Autodesk Inventor part; units mm, degrees
ref_plane "YZ Plane" through (0, 0, 0) normal (1, 0, 0) x (0, 1, 0)
ref_plane "XZ Plane" through (0, 0, 0) normal (0, 1, 0) x (-1, 0, 0)
ref_plane "XY Plane" through (0, 0, 0) normal (0, 0, 1) x (1, 0, 0)
sketch "Sketch1" plane through (0, 0, 0) normal (0, 1, 0) x (-1, 0, 0)
  line L0 (0, 0) -> (105.41, 0)
  line L1 (105.41, 0) -> (105.41, 863.6)
  line L2 (105.41, 863.6) -> (0, 863.6)
  line L3 (0, 863.6) -> (0, 0)
  dimension "d0" = 105.41
  dimension "d1" = 863.6
extrude "Extrusion1" add sketch "Sketch1" along normal blind 12.7
sketch "Sketch2" plane through (0, 12.7, 0) normal (0, 1, 0) x (1, 0, 0)
  line L0 (0, 0) -> (-105.41, 0)
  line L1 (0, 0) -> (-12.7, 0)
  line L2 (-12.7, 0) -> (-12.7, 12.7)
  line L3 (-12.7, 12.7) -> (0, 12.7)
  line L4 (0, 12.7) -> (0, 0)
  line L5 (-105.41, 0) -> (-105.41, -863.6)
  line L6 (0, 12.7) -> (-105.41, 12.7)
  line L7 (-105.41, 12.7) -> (-105.41, 0)
  line L8 (-105.41, 0) -> (0, 0)
  line L9 (0, 0) -> (0, 12.7)
  line L10 (0, -863.6) -> (0, 0)
  line L11 (0, -863.6) -> (-105.41, -863.6)
  line L12 (-105.41, -863.6) -> (-105.41, -876.3)
  line L13 (-105.41, -876.3) -> (0, -876.3)
  line L14 (0, -876.3) -> (0, -863.6)
  line L15 (-105.41, -863.6) -> (-92.71, -863.6)
  line L16 (-92.71, -863.6) -> (-92.71, 12.7)
  line L17 (-92.71, 12.7) -> (-105.41, 12.7)
  line L18 (-105.41, 12.7) -> (-105.41, -863.6)
  line L19 (0, 12.7) -> (-12.7, 12.7)
  line L20 (-12.7, 12.7) -> (-12.7, -876.3)
  line L21 (-12.7, -876.3) -> (0, -876.3)
  line L22 (0, -876.3) -> (0, 12.7)
  point P0 (-12.7, -863.6)
  point P1 (-92.71, 0)
  dimension "d4" = 12.7
  dimension "d5" = 12.7
  dimension "d6" = 12.7
  dimension "d7" = 12.7
  dimension "d8" = 12.7
extrude "Extrusion2" add sketch "Sketch2" along normal blind 95.25 and the other way blind 12.7 contours L10 L11 L20 L0 | L0 L2 L3 L4 | L0 L16 L6 L2 | L14 L13 L20 L11 | L16 L11 L5 L0 | L0 L7 L6 L16 | L20 L13 L12 L11
sketch "Sketch3" plane through (-105.41, 107.95, 876.3) normal (0, 0, 1) x (1, 0, 0)
  line L0 (12.7, -95.25) -> (92.71, -95.25)
  line L1 (12.7, -95.25) -> (12.7, 0)
  line L2 (92.71, -95.25) -> (92.71, 0)
  line L3 (92.71, -95.25) -> (77.47, -95.25)
  line L4 (77.47, -95.25) -> (77.47, -12.7)
  line L5 (77.47, -12.7) -> (92.71, -12.7)
  line L6 (92.71, -12.7) -> (92.71, -95.25)
  line L7 (12.7, -95.25) -> (27.94, -95.25)
  line L8 (27.94, -95.25) -> (27.94, -12.7)
  line L9 (27.94, -12.7) -> (12.7, -12.7)
  line L10 (12.7, -12.7) -> (12.7, -95.25)
  line L11 (27.94, -95.25) -> (34.29, -95.25)
  line L12 (34.29, -95.25) -> (34.29, -12.7)
  line L13 (34.29, -12.7) -> (27.94, -12.7)
  line L14 (27.94, -12.7) -> (27.94, -95.25)
  line L15 (77.47, -95.25) -> (71.12, -95.25)
  line L16 (71.12, -95.25) -> (71.12, -12.7)
  line L17 (71.12, -12.7) -> (77.47, -12.7)
  line L18 (77.47, -12.7) -> (77.47, -95.25)
  line L19 (34.29, -95.25) -> (49.53, -95.25)
  line L20 (49.53, -95.25) -> (49.53, -12.7)
  line L21 (49.53, -12.7) -> (34.29, -12.7)
  line L22 (34.29, -12.7) -> (34.29, -95.25)
  line L23 (71.12, -95.25) -> (55.88, -95.25)
  line L24 (55.88, -95.25) -> (55.88, -12.7)
  line L25 (55.88, -12.7) -> (71.12, -12.7)
  line L26 (71.12, -12.7) -> (71.12, -95.25)
  point P0 (105.41, -107.95)
  dimension "d13" = 15.24
  dimension "d14" = 82.55
  dimension "d15" = 15.24
  dimension "d16" = 6.35
  dimension "d17" = 6.35
  dimension "d18" = 15.24
  dimension "d19" = 15.24
extrude "Extrusion3" cut sketch "Sketch3" against normal blind 95.25 contours L1 L9 L8 L0 | L24 L25 L16 L0 | L12 L21 L20 L0 | L4 L5 L2 L0
sketch "Sketch5" plane through (-105.41, 107.95, 876.3) normal (0, 0, 1) x (1, 0, 0)
  line L0 (71.12, -95.25) -> (55.88, -95.25)
  line L1 (55.88, -95.25) -> (55.88, -12.7)
  line L2 (55.88, -12.7) -> (71.12, -12.7)
  line L3 (71.12, -12.7) -> (71.12, -95.25)
  line L4 (49.53, -95.25) -> (34.29, -95.25)
  line L5 (34.29, -95.25) -> (34.29, -12.7)
  line L6 (34.29, -12.7) -> (49.53, -12.7)
  line L7 (49.53, -12.7) -> (49.53, -95.25)
  line L8 (92.71, -95.25) -> (77.47, -95.25)
  line L9 (77.47, -95.25) -> (77.47, -12.7)
  line L10 (77.47, -12.7) -> (92.71, -12.7)
  line L11 (92.71, -12.7) -> (92.71, -95.25)
  line L12 (27.94, -95.25) -> (12.7, -95.25)
  line L13 (12.7, -95.25) -> (12.7, -12.7)
  line L14 (12.7, -12.7) -> (27.94, -12.7)
  line L15 (27.94, -12.7) -> (27.94, -95.25)
  line L16 (105.41, -107.95) -> (105.41, 0)
  line L17 (0, 0) -> (105.41, 0)
  line L18 (0, -107.95) -> (0, 0)
  line L19 (105.41, -107.95) -> (0, -107.95)
  line L20 (92.71, 0) -> (12.7, 0)
  circle A0 centre (52.705, 26.3525) radius 26.3525
  dimension "d40" = 52.705
extrude "Extrusion4" add sketch "Sketch5" against normal blind 1270 contours A0
sketch "Sketch6" plane through (0, 0, -12.7) normal (1, 0, 0) x (0, 0, -1)
  line L0 (0, 0) -> (-889, 0)
  line L1 (-444.5, 0) -> (-444.5, 160.655)
  line L2 (-889, 160.655) -> (381, 160.655)
  line L3 (-444.5, 160.655) -> (-444.5, 167.005)
  line L4 (-444.5, 0) -> (-444.5, -6.35)
  line L5 (-444.5, 167.005) -> (-428.625, 167.005)
  line L6 (-428.625, 167.005) -> (-460.375, 167.005)
  line L7 (-428.625, 167.005) -> (-460.375, 167.005)
  line L8 (-460.375, 167.005) -> (-460.375, -6.35)
  line L9 (-460.375, -6.35) -> (-428.625, -6.35)
  line L10 (-428.625, -6.35) -> (-428.625, 167.005)
  line L11 (-889, 0) -> (-793.75, 0)
  line L12 (0, 107.95) -> (0, 0)
  line L13 (0, 0) -> (-95.25, 0)
  line L14 (-95.25, 0) -> (-95.25, -6.35)
  line L15 (-793.75, 0) -> (-793.75, -6.35)
  line L16 (-793.75, -6.35) -> (-762, -6.35)
  line L17 (-762, -6.35) -> (-762, 167.005)
  line L18 (-762, 167.005) -> (-793.75, 167.005)
  line L19 (-793.75, 167.005) -> (-793.75, -6.35)
  line L20 (-95.25, -6.35) -> (-127, -6.35)
  line L21 (-127, -6.35) -> (-127, 167.005)
  line L22 (-127, 167.005) -> (-95.25, 167.005)
  line L23 (-95.25, 167.005) -> (-95.25, -6.35)
  line L24 (-111.125, 167.005) -> (-111.125, -6.35)
  line L25 (-777.875, -6.35) -> (-777.875, 167.005)
  line L26 (-777.875, 79.2503) -> (-762, 79.2503)
  line L27 (-111.125, 68.9503) -> (-95.25, 68.9503)
  line L28 (-451.8389, 167.005) -> (-451.8389, 163.0426)
  circle A0 centre (-444.5, 148.7424) radius 10.8761
  circle A1 centre (-444.5, 11.9126) radius 11.9126
  line L29 (-456.4123, 12.0028) -> (-455.3758, 148.8248)
  line L30 (-433.6242, 148.8248) -> (-432.5877, 12.0028)
  line L31 (-127, 12.7) -> (-139.7, 12.7)
  line L32 (-139.7, 12.7) -> (-165.1, 12.7)
  line L33 (-460.375, 21.426) -> (-473.075, 21.426)
  line L34 (0, 107.95) -> (-889, 107.95)
  line L35 (-524.7767, 107.95) -> (-524.7767, 0)
  line L36 (-524.7767, 53.975) -> (-485.775, 53.975)
  circle A2 centre (-485.775, 53.975) radius 12.7
  line L37 (-498.475, 0) -> (-498.475, -3.175)
  line L38 (-498.475, -3.175) -> (-473.075, -3.175)
  line L39 (-473.075, -3.175) -> (-473.075, 53.975)
  line L40 (-498.475, 53.975) -> (-498.475, 0)
  line L41 (-694.0635, 0) -> (-694.0635, 19.05)
  line L42 (-762, 19.05) -> (-571.5, 19.05)
  line L43 (-687.1312, 19.05) -> (-687.1312, 44.45)
  line L44 (-762, 44.45) -> (-565.15, 44.45)
  line L45 (-571.5, 19.05) -> (-565.15, 44.45)
  point P0 (-12.7, 0)
  dimension "d25" = 6.35
  dimension "d26" = 6.35
  dimension "d27" = 15.875
  dimension "d28" = 31.75
  dimension "d29" = 95.25
  dimension "d30" = 95.25
  dimension "d31" = 6.35
  dimension "d32" = 6.35
  dimension "d33" = 31.75
  dimension "d34" = 31.75
  dimension "d35" = 3.9624
  dimension "d39" = 23.8252
  dimension "d41" = 12.7
  dimension "d42" = 25.4
  dimension "d43" = 12.7
  dimension "d45" = 19.05
  dimension "d46" = 190.5
  dimension "d47" = 25.4
  dimension "d48" = 196.85
sketch "Sketch7" plane through (-105.41, 0, 876.3) normal (0, 0, 1) x (1, 0, 0)
  point P0 (105.41, 0)
extrude "Extrusion5" cut sketch "Sketch6" against normal blind 15.24 contours L42 L17 L44 L43 | L43 L44 L45 L42
sketch "Sketch8" plane through (0, 107.95, 0) normal (0, 1, 0) x (1, 0, 0)
  line L0 (0, -876.3) -> (0, 12.7)
  line L1 (-105.41, 12.7) -> (-105.41, -876.3)
  line L2 (0, 12.7) -> (-105.41, 12.7)
  line L3 (-105.41, 12.7) -> (-105.41, -876.3)
  line L4 (-105.41, -876.3) -> (0, -876.3)
  line L5 (0, -876.3) -> (0, 12.7)
  point P0 (0, 0)
extrude "Extrusion6" add sketch "Sketch8" against normal blind 12.7
sketch "Sketch9" plane through (-52.705, 134.3025, 876.3) normal (0, 0, 1) x (1, 0, 0)
  line L0 (-52.705, -26.3525) -> (0, -26.3525)
  line L1 (-39.5109, -26.3525) -> (301.585, -26.3525)
  line L2 (301.585, -26.3525) -> (301.585, 239.994)
  line L3 (301.585, 239.994) -> (-39.5109, 239.994)
  line L4 (-39.5109, 239.994) -> (-39.5109, -26.3525)
  point P0 (52.705, -134.3025)
extrude "Extrusion7" cut sketch "Sketch9" against normal through all
sketch "Sketch10" plane through (-105.41, 0, 876.3) normal (0, 0, 1) x (1, 0, 0)
  point P0 (105.41, 0)
sketch "Sketch11" plane through (0, 107.95, 0) normal (0, 1, 0) x (1, 0, 0)
  line L0 (-105.41, -876.3) -> (0, -876.3)
  line L1 (0, -876.3) -> (0, 12.7)
  line L2 (0, 12.7) -> (-105.41, 12.7)
  line L3 (-105.41, 12.7) -> (-105.41, -876.3)
  line L4 (-92.71, 0) -> (-12.7, 0)
  line L5 (-12.7, 0) -> (-12.7, -863.6)
  line L6 (-12.7, -863.6) -> (-92.71, -863.6)
  line L7 (-92.71, -863.6) -> (-92.71, 0)
  point P0 (0, 0)
  dimension "d55" = 12.7
extrude "Extrusion8" cut sketch "Sketch11" against normal blind 1270 contours L4 L5 L6 L7
sketch "Sketch12" plane through (0, 0, 876.3) normal (1, 0, 0) x (0, 0, -1)
  line L0 (0, 0) -> (0, 107.95)
  line L1 (889, 0) -> (0, 0)
  line L2 (889, 0) -> (889, 107.95)
  line L3 (0, 107.95) -> (889, 107.95)
  line L4 (317.5, 19.05) -> (127, 19.05)
  line L5 (127, 19.05) -> (127, 44.45)
  line L6 (127, 44.45) -> (323.85, 44.45)
  line L7 (323.85, 44.45) -> (317.5, 19.05)
  line L8 (876.3, 95.25) -> (876.3, 12.7)
  line L9 (876.3, 12.7) -> (12.7, 12.7)
  line L10 (12.7, 12.7) -> (12.7, 95.25)
  line L11 (12.7, 95.25) -> (876.3, 95.25)
  point P0 (876.3, 0)
  dimension "d58" = 12.7
extrude "Extrusion9" cut sketch "Sketch12" against normal blind 1270 contours L8 L9 L10 L11
sketch "Sketch13" plane through (-105.41, 19.05, 749.3) normal (-1, 0, 0) x (0, 0, 1)
  line L0 (-207.2337, 33.8649) -> (23.2092, 33.8649)
  line L1 (23.2092, 33.8649) -> (23.2092, -2.854)
  line L2 (23.2092, -2.854) -> (-207.2337, -2.854)
  line L3 (-207.2337, -2.854) -> (-207.2337, 33.8649)
  point P0 (-749.3, -19.05)
extrude "Extrusion10" cut sketch "Sketch13" against normal blind 1270
sketch "Sketch14" plane through (-105.41, 0, 876.3) normal (0, 0, 1) x (1, 0, 0)
  line L0 (105.41, 0) -> (0, 0)
  line L1 (0, 0) -> (106.6554, 0)
  line L2 (106.6554, 0) -> (106.6554, 12.7)
  line L3 (106.6554, 12.7) -> (0, 12.7)
  line L4 (0, 12.7) -> (0, 0)
  line L5 (105.41, 0) -> (105.41, 107.95)
  line L6 (0, 12.7) -> (0, 95.25)
  line L7 (105.41, 107.95) -> (0, 107.95)
  line L8 (0, 107.95) -> (0, 95.25)
  line L9 (0, 95.25) -> (105.41, 95.25)
  line L10 (105.41, 95.25) -> (105.41, 107.95)
  point P0 (105.41, 12.7)
extrude "Extrusion11" add sketch "Sketch14" against normal blind 1270 contours L0 L4 L3 L5 | L9 L8 L7 L5
sketch "Sketch15" plane through (-105.41, 0, 876.3) normal (-1, 0, 0) x (0, 0, 1)
  line L0 (-1270, 0) -> (0, 0)
  line L1 (-888.4017, 0) -> (-1470.844, 0)
  line L2 (-1470.844, 0) -> (-1470.844, 187.8802)
  line L3 (-1470.844, 187.8802) -> (-888.4017, 187.8802)
  line L4 (-888.4017, 187.8802) -> (-888.4017, 0)
  point P0 (-876.3, 0)
extrude "Extrusion12" cut sketch "Sketch15" against normal blind 1270
properties part number "box"
CAD build for the part. Positions are in the model's coordinates, mm. A direction names the side the tool comes from. Give positions to 0.01 mm unless a question says otherwise; leave off trailing zeros. Loops run counter-clockwise (first coordinate to the right, second up) from the corner with the lowest first, then second, coordinate; pieces in that order, holes last. Notation, with made-up numbers: M 85,-32.75 L 100,-32.75 A17 cw 100,-6.75 Z; hole C -22.75,79.25 d8. An arc over 180 degrees is marked long. One line per question, with ' | ' between items. Start each with the question number.
1. Probe L1, parallel to Y at x = -58.5, z = 817; L2, parallel to Z at x = -32, y = 43; L3, parallel to Z at x = -69.5, y = 55. List the from-to ranges inside material, lowest first. Write a range as from..to.
2. Saw through at A-A on z = 65. Give the cut face in (x, y), plus the area to 3 significant figures.
3. Saw through at B-B on y = 83. Give the cut face in (x, z), plus the area to 3 significant figures.
4. Two-plate mould, pull along Y, no slides. Class faces 3 (the face through (-53, 107.95, 426)), 4 (the face through (-52, 95.25, 444)), 5 (the face through (-105.41, 10, 430)): pulls with the +Y half, pulls with the -Y half, needs draft (parallel to the pull), parting line crosses it, or undercut.
5. 3-axis set-ups, long thin cutter, end or side, ignore diameter. For faces 1 (the face through (-53, 55, 0)), 2 (the face through (-53, 55, -12.102)): which of +Z, -Z, +X, -X, +Y, -Y reach the whole face in a straight line?
6. Flat gauge pin, fed straight in: pin 1 (2 mm diameter, centred on x = -46.5, y = 63, fed in from +Z). Where does the tip first touch, or does it go through?
Result sheet:
1) L1: y = 0..12.7, 95.25..107.95 | L2: z = -12.1..0, 863.6..876.3 | L3: z = -12.1..0
2) outline: M -105.41,0 L 0,0 L 0,12.7 L -105.41,12.7 Z; M -105.41,95.25 L 0,95.25 L 0,107.95 L -105.41,107.95 Z | area: 2,680 mm^2
3) outline: M -105.41,-12.1 L 0,-12.1 L 0,0 L -105.41,0 Z; M -105.41,863.6 L -92.71,863.6 L -92.71,876.3 L -105.41,876.3 Z; M -77.47,863.6 L -71.12,863.6 L -71.12,876.3 L -77.47,876.3 Z; M -55.88,863.6 L -49.53,863.6 L -49.53,876.3 L -55.88,876.3 Z; M -34.29,863.6 L -27.94,863.6 L -27.94,876.3 L -34.29,876.3 Z; M -12.7,863.6 L 0,863.6 L 0,876.3 L -12.7,876.3 Z | area: 1,840 mm^2
4) face 3: pulls with the +Y half | face 4: undercut | face 5: needs draft
5) face 1: +X, -X | face 2: -Z, +X, -X, +Y, -Y
6) pin 1: stops at z = 0
